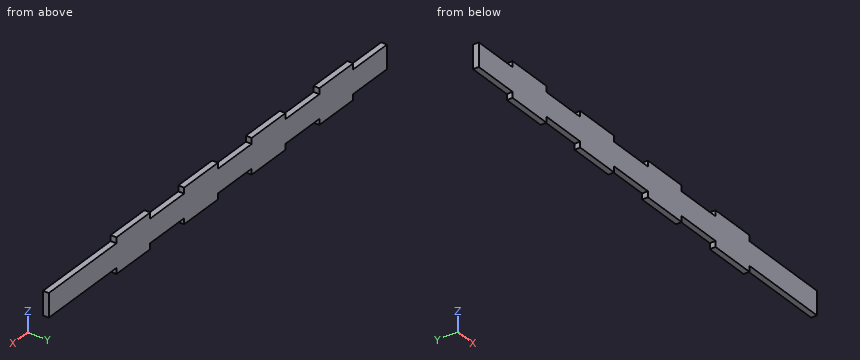
from build123d import *

# Parameters (mm, degrees)
BOSS_EXTRUDE1_DEPTH = 1.5875


with BuildPart() as part:
    # Sketch1 → Boss-Extrude1 (new body, symmetric)
    with BuildSketch(Plane(origin=(0, 0, 0), x_dir=(1, 0, 0), z_dir=(0, 1, 0))):
        Polygon((-114.3, 6.5), (-114.3, -6.5), (-88.9, -6.5), (-88.9, -9.675), (-63.5, -9.675), (-63.5, -6.5), (-38.1, -6.5), (-38.1, -9.675), (-12.7, -9.675), (-12.7, -6.5), (12.7, -6.5), (12.7, -9.675), (38.1, -9.675), (38.1, -6.5), (63.5, -6.5), (63.5, -9.675), (88.9, -9.675), (88.9, -6.5), (139.7, -6.5), (139.7, 6.5), (88.9, 6.5), (88.9, 9.675), (63.5, 9.675), (63.5, 6.5), (38.1, 6.5), (38.1, 9.675), (12.7, 9.675), (12.7, 6.5), (-12.7, 6.5), (-12.7, 9.675), (-38.1, 9.675), (-38.1, 6.5), (-63.5, 6.5), (-63.5, 9.675), (-88.9, 9.675), (-88.9, 6.5), align=None)
    extrude(amount=BOSS_EXTRUDE1_DEPTH, both=True)


solid = part.part
The listing builds one solid part. Answer for the finished solid, in the listing's coordinates (mm). Round coordinates to 2 decimals unless told otherwise and drop trailing zeros. Order: outer loops, then holes, each group sorted by start corner. A loop starts at its lowest first (then second) coordinate and runs counter-clockwise, first axis right, second up. Notation, with made-up numbers: (-10.5, 10) -> (46.5, 10) arc R37 cw to (46.5, 49) -> close; hole circle Ø5 at (-33, -37.5). An arc over 180 degrees is marked (long way). One line per item, written item: value.
Item 1: Find section A-A, the plane x = 50. Give the vertices of the cut face in (y, z), then the cut area to 3 significant figures.
Taken from the geometry:
outline: (-1.59, -6.5) -> (1.59, -6.5) -> (1.59, 6.5) -> (-1.59, 6.5) -> close
area: 41.3 mm2
Item 2: Given P1, Ø1, axis at x = -3, y = 0.5, coming from the -Z side; P2, Ø1.6, axis at x = -4.5, y = 0, coming from the +Z side; P3, Ø1, axis at y = -0.5, z = -9, coming from the -X side, each flat-ended and moving along its own axis, determine where each tip first touches the part or whether it passes through.
Taken from the geometry:
P1: stops at z = -6.5
P2: stops at z = 6.5
P3: stops at x = -88.9
Item 3: Straight lines are drawn through the part: L1, parallel to X at y = 1.45, z = 8.5; L2, parallel to Z at x = 5.5, y = -0.1. For each, find the intervals that lie inside material, in ascending order.
Taken from the geometry:
L1: x = -88.9 to -63.5, -38.1 to -12.7, 12.7 to 38.1, 63.5 to 88.9
L2: z = -6.5 to 6.5
